Autodesk Inventor part; units mm, degrees
ref_plane "YZ Plane" through (0, 0, 0) normal (1, 0, 0) x (0, 1, 0)
ref_plane "XZ Plane" through (0, 0, 0) normal (0, 1, 0) x (-1, 0, 0)
ref_plane "XY Plane" through (0, 0, 0) normal (0, 0, 1) x (1, 0, 0)
sketch "Esboço1" plane through (0, 0, 0) normal (0, 0, 1) x (1, 0, 0)
  arc A0 (19, -10) -> (20, -9) centre (19, -9) ccw
  line L0 (20, -4.8) -> (20, -9)
  line L1 (18.2, -3) -> (20, -4.8)
  line L2 (18.2, -5.5) -> (18.2, -3)
  line L3 (16.5607, -5.5) -> (18.2, -5.5)
  line L4 (14, -2.9393) -> (16.5607, -5.5)
  line L5 (14, -0.3) -> (14, -2.9393)
  line L6 (13.7, 0) -> (14, -0.3)
  line L7 (14, 0.3) -> (13.7, 0)
  line L8 (14, 2.9393) -> (14, 0.3)
  line L9 (16.5607, 5.5) -> (14, 2.9393)
  line L10 (18.2, 5.5) -> (16.5607, 5.5)
  line L11 (18.2, 3) -> (18.2, 5.5)
  line L12 (20, 4.8) -> (18.2, 3)
  line L13 (20, 9) -> (20, 4.8)
  arc A1 (20, 9) -> (19, 10) centre (19, 9) ccw
  line L14 (14.8, 10) -> (19, 10)
  line L15 (13, 8.2) -> (14.8, 10)
  line L16 (15.5, 8.2) -> (13, 8.2)
  line L17 (15.5, 6.5607) -> (15.5, 8.2)
  line L18 (12.9393, 4) -> (15.5, 6.5607)
  line L19 (10.3, 4) -> (12.9393, 4)
  line L20 (10, 3.7) -> (10.3, 4)
  line L21 (9.7, 4) -> (10, 3.7)
  line L22 (7.0607, 4) -> (9.7, 4)
  line L23 (4.5, 6.5607) -> (7.0607, 4)
  line L24 (4.5, 8.2) -> (4.5, 6.5607)
  line L25 (7, 8.2) -> (4.5, 8.2)
  line L26 (5.2, 10) -> (7, 8.2)
  line L27 (-5.2, 10) -> (5.2, 10)
  line L28 (-7, 8.2) -> (-5.2, 10)
  line L29 (-4.5, 8.2) -> (-7, 8.2)
  line L30 (-4.5, 6.5607) -> (-4.5, 8.2)
  line L31 (-7.0607, 4) -> (-4.5, 6.5607)
  line L32 (-9.7, 4) -> (-7.0607, 4)
  line L33 (-10, 3.7) -> (-9.7, 4)
  line L34 (-10.3, 4) -> (-10, 3.7)
  line L35 (-12.9393, 4) -> (-10.3, 4)
  line L36 (-15.5, 6.5607) -> (-12.9393, 4)
  line L37 (-15.5, 8.2) -> (-15.5, 6.5607)
  line L38 (-13, 8.2) -> (-15.5, 8.2)
  line L39 (-14.8, 10) -> (-13, 8.2)
  line L40 (-19, 10) -> (-14.8, 10)
  arc A2 (-19, 10) -> (-20, 9) centre (-19, 9) ccw
  line L41 (-20, 4.8) -> (-20, 9)
  line L42 (-18.2, 3) -> (-20, 4.8)
  line L43 (-18.2, 5.5) -> (-18.2, 3)
  line L44 (-16.5607, 5.5) -> (-18.2, 5.5)
  line L45 (-14, 2.9393) -> (-16.5607, 5.5)
  line L46 (-14, 0.3) -> (-14, 2.9393)
  line L47 (-13.7, 0) -> (-14, 0.3)
  line L48 (-14, -0.3) -> (-13.7, 0)
  line L49 (-14, -2.9393) -> (-14, -0.3)
  line L50 (-16.5607, -5.5) -> (-14, -2.9393)
  line L51 (-18.2, -5.5) -> (-16.5607, -5.5)
  line L52 (-18.2, -3) -> (-18.2, -5.5)
  line L53 (-20, -4.8) -> (-18.2, -3)
  line L54 (-20, -9) -> (-20, -4.8)
  arc A3 (-20, -9) -> (-19, -10) centre (-19, -9) ccw
  line L55 (-14.8, -10) -> (-19, -10)
  line L56 (-13, -8.2) -> (-14.8, -10)
  line L57 (-15.5, -8.2) -> (-13, -8.2)
  line L58 (-15.5, -6.5607) -> (-15.5, -8.2)
  line L59 (-12.9393, -4) -> (-15.5, -6.5607)
  line L60 (-10.3, -4) -> (-12.9393, -4)
  line L61 (-10, -3.7) -> (-10.3, -4)
  line L62 (-9.7, -4) -> (-10, -3.7)
  line L63 (-7.0607, -4) -> (-9.7, -4)
  line L64 (-4.5, -6.5607) -> (-7.0607, -4)
  line L65 (-4.5, -8.2) -> (-4.5, -6.5607)
  line L66 (-7, -8.2) -> (-4.5, -8.2)
  line L67 (-5.2, -10) -> (-7, -8.2)
  line L68 (5.2, -10) -> (-5.2, -10)
  line L69 (7, -8.2) -> (5.2, -10)
  line L70 (4.5, -8.2) -> (7, -8.2)
  line L71 (4.5, -6.5607) -> (4.5, -8.2)
  line L72 (7.0607, -4) -> (4.5, -6.5607)
  line L73 (9.7, -4) -> (7.0607, -4)
  line L74 (10, -3.7) -> (9.7, -4)
  line L75 (10.3, -4) -> (10, -3.7)
  line L76 (12.9393, -4) -> (10.3, -4)
  line L77 (15.5, -6.5607) -> (12.9393, -4)
  line L78 (15.5, -8.2) -> (15.5, -6.5607)
  line L79 (13, -8.2) -> (15.5, -8.2)
  line L80 (14.8, -10) -> (13, -8.2)
  line L81 (19, -10) -> (14.8, -10)
  line L82 (-2.7, 8.2) -> (2.7, 8.2)
  line L83 (2.7, 8.2) -> (2.7, 6.2393)
  line L84 (2.7, 6.2393) -> (6, 2.9393)
  line L85 (6, 2.9393) -> (6, -2.9393)
  line L86 (6, -2.9393) -> (2.7, -6.2393)
  line L87 (2.7, -6.2393) -> (2.7, -8.2)
  line L88 (2.7, -8.2) -> (-2.7, -8.2)
  line L89 (-2.7, -8.2) -> (-2.7, -6.2393)
  line L90 (-2.7, -6.2393) -> (-6, -2.9393)
  line L91 (-6, -2.9393) -> (-6, 2.9393)
  line L92 (-6, 2.9393) -> (-2.7, 6.2393)
  line L93 (-2.7, 6.2393) -> (-2.7, 8.2)
  circle A4 centre (10, 0) radius 2.5
  circle A5 centre (-10, 0) radius 2.5
  point P0 (0, 0)
  point P1 (0, 0)
extrude "Extrusão1" add sketch "Esboço1" along normal blind 1054
properties part number "PERFIL_ESTRUTURAL_20X40_MESA"
Design review of the part built by this model. Coordinates are the model's own, in mm. Give positions to 0.01 mm unless a question says otherwise; leave off trailing zeros. Write item = value, one per line.
Q1. To check wall thickness, follow line 1 (X direction, y = 9.25, z = 946.5); line 2 (X direction, y = 7.25, z = 273); line 3 (Y direction, x = -10, z = 352.5). State the ranges of each line that lie inside material, in increasing order. Write a range as [from, to].
Output values:
line_1 = [-19.97, -14.05], [-5.95, 5.95], [14.05, 19.97]
line_2 = [-20, -15.5], [-4.5, -2.7], [2.7, 4.5], [15.5, 20]
line_3 = [-3.7, -2.5], [2.5, 3.7]
Q2. We need section A-A (z = 174). Count the separate pieces of the cut face and the enclosed holes in it, plus the area to 3 significant figures.
Output values:
separate_pieces = 1
enclosed_holes = 3
area = 288 mm^2
Q3. Insertion check: pin 1 (6 mm diameter, centred on x = 8.5, z = 807, fed in from -Y); pin 2 (1.3 mm diameter, centred on x = -12, z = 520.5, fed in from -Y); pin 3 (6.5 mm diameter, centred on y = -0.5, z = 670.5, fed in from +X). Each pin has a flat end and moves straight along its axis. Give the tip position at first contact, or say it passes through.
Output values:
pin_1 = -9.7
pin_2 = -4
pin_3 = 18.95
